Verification items for the finished model (mm, model axes). Face numbers are marked on the shaded views. A direction names the side the tool comes from. Round coordinates to 2 decimals unless told otherwise and drop trailing zeros. Order: outer loops, then holes, each group sorted by start corner. A loop starts at its lowest first (then second) coordinate and runs counter-clockwise, first axis right, second up. Notation, with made-up numbers: M -35,-10.5 L -18,-10.5 A23 cw -18,7.5 Z; hole C 73.5,3 d8. An arc over 180 degrees is marked long. Answer as a JSON object with one key per item and string values. Group by question number.
```python
from build123d import *

# Parameters (mm, degrees)
SKETCH010_R             = 7.5
SKETCH010_R_2           = 3.05
PAD002_DEPTH            = 9.5
SKETCH009_R             = 6.5
PAD003_DEPTH            = 1.1
FILLET001_R             = 1
SKETCH011_R             = 1.5
POCKET001_DEPTH         = 5
BODY001_PLACEMENT_ANGLE = 90


with BuildPart() as part:
    # Sketch010 → Pad002 (new body)
    with BuildSketch(Plane.XY):
        Circle(SKETCH010_R)
        Circle(SKETCH010_R_2, mode=Mode.SUBTRACT)
    extrude(amount=PAD002_DEPTH)

    # Sketch009 (on Face4 of Pad002) → Pad003 (join)
    with BuildSketch(Plane.XY.offset(9.5)):
        Circle(SKETCH009_R)
    extrude(amount=PAD003_DEPTH)

    # Fillet001
    fillet001_edges = [part.edges().sort_by_distance(p)[0] for p in [
        (-6.5, 0, 10.6),
    ]]
    fillet(fillet001_edges, radius=FILLET001_R)

    # Sketch011 (on DatumPlane) → Pocket001 (cut)
    with BuildSketch(Plane(origin=(-8, 0, 4.75), x_dir=(0, 0, 1), z_dir=(-1, 0, 0))):
        Circle(SKETCH011_R)
    extrude(amount=-POCKET001_DEPTH, mode=Mode.SUBTRACT)


with BuildPart() as part_1:
    # Body001 placement: moved
    add(part.part.moved(Location((41, 28, 28))).rotate(Axis((41, 28, 28), (0, 1, 0)), BODY001_PLACEMENT_ANGLE))


solid = part_1.part
```
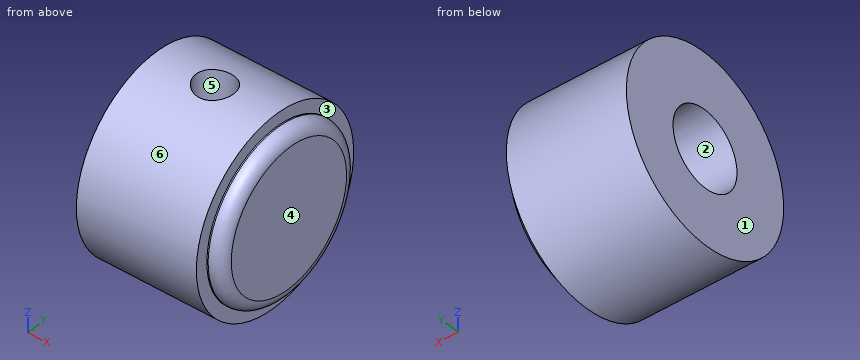
Q1. Gauge pin test, flat ends, axial feed: pin 1 Ø5 at (x, y) = (42.5, 32.5) entering from -Z; pin 2 Ø1.5 at (x, z) = (43, 25.5) entering from -Y; pin 3 Ø0.8 at (x, y) = (45.5, 29) entering from +Z. Record the tip position at first contact, or that the pin passes through.
Q2. Cross-section at A-A, the plane y = 28. Record the cut outline in (x, z), then the cut area to 3 significant figures.
Q3. Cross-section at D-D, the plane x = 44.75. Record the cut outline in (y, z).
Q4. Thickness scan on line 1 (X direction, y = 21.5, z = 31); line 2 (Y direction, x = 45.75, z = 34.75); line 3 (Y direction, x = 46, z = 28). Record the ranges inside material, lowest first. Write a range as from..to.
Q5. Cross-section at C-C, the plane x = 49.75. Record the cut outline in (y, z).
Q6. Release check for a two-part mould opening along Y. For the marked faces 4, 5 and 6 record: released by +Y, released by -Y, zero draft, split by the parting line, or undercut.
Q7. Tool access check on the marked faces 1, 2 and 3. Record the directions out of +Z, -Z, +X, -X, +Y, -Y that give a thin tool (end or side, any length) a straight path to the whole face; none if there is none.
Q8. Cross-section at B-B, the plane z = 28. Record the cut outline in (x, y), then the cut area to 3 significant figures.
Conclusion:
{
 "1": {"pin 1": "z = 20.77", "pin 2": "y = 20.71", "pin 3": "z = 31"},
 "2": {"outline": "M 41,20.5 L 50.5,20.5 L 50.5,21.5 L 50.6,21.5 A1 ccw 51.6,22.5 L 51.6,33.5 A1 ccw 50.6,34.5 L 50.5,34.5 L 50.5,35.5 L 47.25,35.5 L 47.25,31.05 L 50.5,31.05 L 50.5,24.95 L 41,24.95 Z; M 41,31.05 L 44.25,31.05 L 44.25,35.5 L 41,35.5 Z", "area": "85.1 mm2"},
 "3": {"outline": "M 26.88,31 L 26.88,35.42 A7.5 ccw long 29.12,35.42 L 29.12,31 L 28.55,31 A3.05 cw long 27.45,31 Z"},
 "4": {"line 1": "41..50.5", "line 2": "24.73..26.5, 29.5..31.27", "line 3": "20.5..24.95, 31.05..35.5"},
 "5": {"outline": "C 28,28 d15; hole C 28,28 d6.1"},
 "6": {"face 4": "zero draft", "face 5": "undercut", "face 6": "split by the parting line"},
 "7": {"face 1": "+Z, -Z, -X, +Y, -Y", "face 2": "-X", "face 3": "+X"},
 "8": {"outline": "M 41,20.5 L 50.5,20.5 L 50.5,21.5 L 50.6,21.5 A1 ccw 51.6,22.5 L 51.6,33.5 A1 ccw 50.6,34.5 L 50.5,34.5 L 50.5,35.5 L 41,35.5 L 41,31.05 L 50.5,31.05 L 50.5,24.95 L 41,24.95 Z", "area": "98.4 mm2"}
}
